Verification items for the finished model (mm, model axes). Round coordinates to 2 decimals unless told otherwise and drop trailing zeros. Write each loop counter-clockwise with the first axis right and the second up, starting at its lowest first coordinate (ties: lowest second). Pieces come first, ordered by that corner, then holes. Notation, with made-up numbers: (26.25, -2.5) - (50.25, -2.5) arc R20 cw to (50.25, 7.5) - close; hole circle Ø4 at (47, 60). An arc over 180 degrees is marked (long way). Answer as a JSON object with one key per item and string values. Group by question number.
1) Section check A-A (y = -1.5). Enter the section's corners in (x, z), then the cut area to 3 significant figures.
2) Go/stop test with flat-tipped pins: pin 1 Ø6 at (y, z) = (-1, 133.5) entering from -X; pin 2 Ø5 at (y, z) = (3.5, 281.5) entering from -X; pin 3 Ø1 at (y, z) = (0.5, 238.5) entering from -X. Record where each tip stops, or that it passes through.
3) Section check B-B (z = 156). Enter the section's corners in (x, y).
4) Thickness scan on line 1 (X direction, y = 2, z = 157.5); line 2 (X direction, y = -0.75, z = 118.5). Record the ranges inside material, lowest first.
5) Section check C-C (x = 98). Enter the section's corners in (y, z).
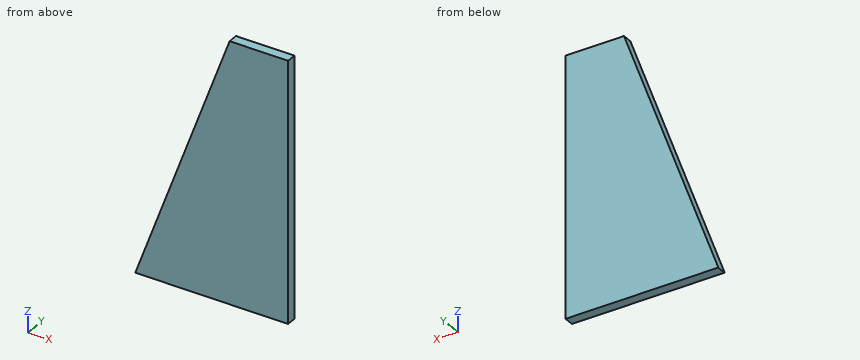
```python
from build123d import *

# Parameters (mm, degrees)
PAD_DEPTH = 6.5


with BuildPart() as part:
    # Sketch → Pad (new body, symmetric)
    with BuildSketch(Plane.XZ):
        Polygon((0, 0), (200, 0), (200, 340), (123.385909, 340), (0, 1), align=None)
    extrude(amount=PAD_DEPTH, both=True)


solid = part.part
```
Returned:
{
 "1": {"outline": "(0, 0) - (200, 0) - (200, 340) - (123.39, 340) - (0, 1) - close", "area": "47,100 mm2"},
 "2": {"pin 1": "x = 47.13", "pin 2": "x = 101.18", "pin 3": "x = 86.26"},
 "3": {"outline": "(56.42, -6.5) - (200, -6.5) - (200, 6.5) - (56.42, 6.5) - close"},
 "4": {"line 1": "56.96 to 200", "line 2": "42.77 to 200"},
 "5": {"outline": "(-6.5, 0) - (6.5, 0) - (6.5, 270.25) - (-6.5, 270.25) - close"}
}
